from build123d import *

# Parameters (mm, degrees)
RESSALTO_EXTRUS_O1_DEPTH   = 5
ESBO_O3_R                  = 12.5
RESSALTO_EXTRUS_O2_DEPTH   = 7
CORTE_EXTRUS_O1_DEPTH      = 30.100324457
CORTE_EXTRUS_O1_DEPTH_BACK = 30.100324457
ESBO_O2_R                  = 6
ESBO_O2_R_2                = 2.75
FILETE8_R                  = 5.5
FILETE9_R                  = 5.5
FILETE10_R                 = 5.5
FILETE11_R                 = 5.5
CORTE_EXTRUS_O2_DEPTH      = 31.689230742
CORTE_EXTRUS_O2_DEPTH_BACK = 31.689230742
ESBO_O4_W                  = 1.736979024
ESBO_O4_H                  = 15.670956688


with BuildPart() as part:
    # Ressalto-extrusão1: read off the stored shape, not the designer's step
    # Ressalto-extrusão1 outline → Ressalto-extrusão1 (new body)
    with BuildSketch(Plane.XY):
        Polygon((4.775767162, -12.578134648), (23.5, -2.5), (23.5, 2.5), (3.728917801, 12.329043312), (-3.728917801, 12.329043312), (-23.5, 2.5), (-23.5, -2.5), (-4.775767162, -12.578134648), (-4.775767162, -15.670956688), (-0.868489512, -15.670956688), (-0.868489512, 0), (0.868489512, 0), (0.868489512, -15.670956688), (4.775767162, -15.670956688), align=None)
    extrude(amount=RESSALTO_EXTRUS_O1_DEPTH)

    # Esboço3 → Ressalto-extrusão2 (add)
    with BuildSketch(Plane.XY.offset(5)):
        with Locations(Location((0, 0, 0), (0, 0, 99.486846806))):
            Circle(ESBO_O3_R)
    extrude(amount=RESSALTO_EXTRUS_O2_DEPTH)

    # Esboço2 → Corte-extrusão1 (cut, two sides: drawn at the far end of the back side and taken through both)
    with BuildSketch(Plane.XY.offset(5).offset(-CORTE_EXTRUS_O1_DEPTH_BACK)):
        Circle(ESBO_O2_R)
        with Locations((-18, 0)):
            Circle(ESBO_O2_R_2)
        with Locations((18, 0)):
            Circle(ESBO_O2_R_2)
    extrude(amount=CORTE_EXTRUS_O1_DEPTH + CORTE_EXTRUS_O1_DEPTH_BACK, mode=Mode.SUBTRACT)

    # Filete8
    filete8_edges = [part.edges().sort_by_distance(p)[0] for p in [
        (-23.5, 2.5, 2.5),
    ]]
    fillet(filete8_edges, radius=FILETE8_R)

    # Filete9
    # the kernel refuses this fillet: 5.5 mm, written as the material it takes off along each edge
    with BuildSketch(Plane(origin=(-23.5, -2.5, -7.284114841), x_dir=(1.1558918030709584e-12, 1.0, 0), z_dir=(0, 0, 1))) as filete9_piece_1:
        with BuildLine():
            CenterArc((3.462119709, -5.172336006), FILETE9_R, 109.876993247, 41.832083594)
            Line((-1.380918754, -2.565618062), (-1.477779523, -2.513483703))
            Line((-1.477779523, -2.513483703), (-0.096860769, 0.052134359))
            Line((-0.096860769, 0.052134359), (0, 0.11))
            ThreePointArc((0, 0.11), (0.796054475, 0.11), (1.554708735, 0.10344672))
            Line((1.554708735, 0.10344672), (1.592108951, 0))
        make_face()
    extrude(amount=19.568229683, mode=Mode.SUBTRACT)

    # Filete10
    filete10_edges = [part.edges().sort_by_distance(p)[0] for p in [
        (23.5, 2.5, 2.5),
    ]]
    fillet(filete10_edges, radius=FILETE10_R)

    # Filete11
    # the kernel refuses this fillet: 5.5 mm, written as the material it takes off along each edge
    with BuildSketch(Plane(origin=(23.5, -2.5, -7.284114841), x_dir=(-1.1603547057855156e-12, 1.0, 0), z_dir=(0, 0, 1))) as filete11_piece_1:
        with BuildLine():
            CenterArc((3.462119709, 5.172336006), FILETE11_R, 208.290923159, 41.832083594)
            Line((-1.380918754, 2.565618062), (-1.477779523, 2.513483703))
            Line((-1.477779523, 2.513483703), (-0.096860769, -0.052134359))
            Line((-0.096860769, -0.052134359), (0, -0.11))
            ThreePointArc((0, -0.11), (0.796054475, -0.11), (1.554708735, -0.10344672))
            Line((1.554708735, -0.10344672), (1.592108951, 0))
        make_face()
    extrude(amount=19.568229683, mode=Mode.SUBTRACT)

    # Esboço4 → Corte-extrusão2 (cut, two sides: drawn at the far end of the back side and taken through both)
    with BuildSketch(Plane.XY.offset(12).offset(-CORTE_EXTRUS_O2_DEPTH_BACK)):
        with Locations((0, -7.835478344)):
            Rectangle(ESBO_O4_W, ESBO_O4_H)
    extrude(amount=CORTE_EXTRUS_O2_DEPTH + CORTE_EXTRUS_O2_DEPTH_BACK, mode=Mode.SUBTRACT)


solid = part.part
Read the model definition and answer for the solid it produces. Units are mm, in the model's axes. A direction names the side the tool comes from. Coordinates: 2 decimals unless noted, no trailing zeros. Write each loop counter-clockwise with the first axis right and the second up, starting at its lowest first coordinate (ties: lowest second). Pieces come first, ordered by that corner, then holes. Notation, with made-up numbers: (33, 34.5) -> (62, 34.5) arc R16 cw to (62, 52.5) -> close; hole circle Ø2 at (16, 19). An arc over 180 degrees is marked (long way). Return JSON: item names as keys, results as strings.
(1) Each of these flat-tipped pins is pushed along its axis until it touches: P1, Ø1.5, axis at y = -14, z = 1.5, coming from the -X side; P2, Ø6, axis at y = -0.5, z = 11, coming from the -X side; P3, Ø0.9, axis at y = -14, z = 3, coming from the +X side; P4, Ø9.5, axis at x = 0, y = 0, coming from the +Z side. Where does it stop, or does it pass through?
Answers below:
{"P1": "x = -4.78", "P2": "x = -12.5", "P3": "x = 4.78", "P4": "through"}
(2) The part is cut by section A-A on z = 1.5. Give the vertices of the cut face in (x, y).
Answers below:
{"outline": "(-23.5, -0.91) arc R5.5 ccw to (-20.93, -3.88) -> (-4.78, -12.58) -> (-4.78, -15.67) -> (-0.87, -15.67) -> (-0.87, -5.94) arc R6 cw (long way) to (0.87, -5.94) -> (0.87, -15.67) -> (4.78, -15.67) -> (4.78, -12.58) -> (20.93, -3.88) arc R5.5 ccw to (23.5, -0.91) arc R5.5 ccw to (20.45, 4.02) -> (3.73, 12.33) -> (-3.73, 12.33) -> (-20.45, 4.02) arc R5.5 ccw to start; hole circle Ø5.5 at (-18, 0); hole circle Ø5.5 at (18, 0)"}
(3) Consider line 1 along X through (y, z) = (-1, 1.5); line 2 along Z through (x, y) = (13, 7.5); line 3 along X through (y, z) = (0, 3). Determine where each line is inside the solid, lowest interval first. Write a range as from..to.
Answers below:
{"line 1": "-23.47..-20.56, -15.44..-5.92, 5.92..15.44, 20.56..23.47", "line 2": "0..5", "line 3": "-23.42..-20.75, -15.25..-6, 6..15.25, 20.75..23.42"}
(4) The part is cut by section D-D on x = -7. Give the vertices of the cut face in (y, z).
Answers below:
{"outline": "(-11.38, 0) -> (10.7, 0) -> (10.7, 5) -> (10.36, 5) -> (10.36, 12) -> (-10.36, 12) -> (-10.36, 5) -> (-11.38, 5) -> close"}
(5) The part is cut by section B-B on x = 19.5. Give the vertices of the cut face in (y, z).
Answers below:
{"outline": "(-4.65, 0) -> (-2.3, 0) -> (-2.3, 5) -> (-4.65, 5) -> close; (2.3, 0) -> (4.49, 0) -> (4.49, 5) -> (2.3, 5) -> close"}
(6) For a pull along Y with two mould halves and no side action, classify faces 5 (the flat face through (12.74, -8.29, 2.46)), 6 (the cylindrical face through (0, 6, 6)), 7 (the flat face through (5, 5, 0)) as pulls with the +Y half, pulls with the -Y half, needs draft (parallel to the pull), parting line crosses it, or undercut.
Answers below:
{"face 5": "pulls with the -Y half", "face 6": "undercut", "face 7": "needs draft"}
(7) The part is cut by section C-C on y = 0. Give the vertices of the cut face in (x, z), then the cut area to 3 significant figures.
Answers below:
{"outline": "(-23.42, 0) -> (-20.75, 0) -> (-20.75, 5) -> (-23.42, 5) -> close; (-15.25, 0) -> (-6, 0) -> (-6, 12) -> (-12.5, 12) -> (-12.5, 5) -> (-15.25, 5) -> close; (6, 0) -> (15.25, 0) -> (15.25, 5) -> (12.5, 5) -> (12.5, 12) -> (6, 12) -> close; (20.75, 0) -> (23.42, 0) -> (23.42, 5) -> (20.75, 5) -> close", "area": "210 mm^2"}
(8) Which of the six approach directions +Z, -Z, +X, -X, +Y, -Y give full straight-line access (tool end or side, diameter ignored) to faces 1 (the cylindrical face through (0.54, 12.49, 8.45)), 2 (the flat face through (-4.776, -14, 2)), 3 (the flat face through (0.868, -10, 6)), 4 (the flat face through (4.776, -14, 2))?
Answers below:
{"face 1": "+Z", "face 2": "+Z, -Z, -X, -Y", "face 3": "+Z, -Z, -Y", "face 4": "+Z, -Z, +X, -Y"}
